Check sheet for the modelled part. Datum: model origin and axes. Units: mm. Coordinates: 2 decimals unless noted, no trailing zeros. Order: outer loops, then holes, each group sorted by start corner. A loop starts at its lowest first (then second) coordinate and runs counter-clockwise, first axis right, second up.
from build123d import *


with BuildPart() as part:
    # Esboço1 → Revolução1 (revolve)
    with BuildSketch(Plane.XY, mode=Mode.PRIVATE) as revolu_o1_sk:
        with BuildLine():
            Line((0, 0.4), (0.7, 0.4))
            Line((0.7, 0.4), (0.7, 0.484529946))
            Line((0.7, 0.484529946), (0.9, 0.6))
            Line((0.9, 0.6), (2.2, 0.6))
            Line((2.2, 0.6), (3.4, 1.2))
            Line((3.4, 1.2), (3.6, 1.2))
            Line((3.6, 1.2), (3.6, 0.99))
            Line((3.6, 0.99), (7.35, 0.99))
            Line((7.35, 0.99), (7.6, 0.845662433))
            Line((7.6, 0.845662433), (7.6, 0.4))
            Line((7.6, 0.4), (31.895599944, 0.4))
            Line((31.895599944, 0.4), (34.437226116, 0.177636523))
            ThreePointArc((34.437226116, 0.177636523), (34.553152591, 0.120467912), (34.6, 0))
            Line((34.6, 0), (-0.4, 0))
            ThreePointArc((-0.4, 0), (-0.282842712, 0.282842712), (0, 0.4))
        make_face()
    revolve(revolu_o1_sk.sketch.rotate(Axis((-0.4, 0, 0), (1, 0, 0)), 90), axis=Axis((-0.4, 0, 0), (1, 0, 0)))


solid = part.part
(1) Thickness scan on probe 1 along Y at (x, z) = (10, 0.05); probe 2 along Z at (x, y) = (7.5, -0.6); probe 3 along X at (y, z) = (0.1, 0). Record the ranges inside material, lowest first.
Filled in:
probe 1: y = -0.4 to 0.4
probe 2: z = -0.68 to 0.68
probe 3: x = -0.39 to 34.57
(2) Cross-section at B-B (x = 6.5). Enter the section's corners in (y, z).
Filled in:
outline: circle Ø1.98 at (0, 0)
(3) Release check for a two-part mould opening along X. For faces 1 (the cylindrical face through (1.559, -0.506, 0.323)), 2 (the conical face through (2.41, 0.69, -0.15)) record: +X half, -X half, draft (parallel to the pull), parting line (faces both ways), or undercut.
Filled in:
face 1: draft
face 2: -X half
(4) Cross-section at A-A (x = 28). Enter the section's corners in (y, z), and give its area (3 significant figures).
Filled in:
outline: circle Ø0.8 at (0, 0)
area: 0.503 mm2
